Work out the finished part from the listing and answer in its coordinate system (mm). Face numbers are marked on the shaded views. Round coordinates to 2 decimals unless told otherwise and drop trailing zeros. Loops run counter-clockwise (first coordinate to the right, second up) from the corner with the lowest first, then second, coordinate; pieces in that order, holes last. Notation, with made-up numbers: (61, 53.5) -> (89, 53.5) arc R21 ccw to (89, 82.5) -> close; hole circle Ø1 at (-39, -37.5). An arc over 180 degrees is marked (long way). Write item = value, one per line. Start each with the question number.
```python
from build123d import *

# Parameters (mm, degrees)
F0_W     = 900
F0_H     = 2000
F1_DEPTH = 270
F2_R     = 20
F3_W     = 80
F3_H     = 80
F4_DEPTH = 100


with BuildPart() as f1:
    # F0 (on Top) → F1 (new body)
    with BuildSketch(Plane.XY):
        Rectangle(F0_W, F0_H)
    extrude(amount=F1_DEPTH)

    # F2
    f2_edges = [f1.edges().sort_by_distance(p)[0] for p in [
        (-450, 0, 270),
        (0, 1000, 270),
        (450, 0, 270),
        (0, -1000, 270),
        (450, -1000, 135),
        (450, 1000, 135),
        (-450, 1000, 135),
        (-450, -1000, 135),
    ]]
    fillet(f2_edges, radius=F2_R)

    # F3 (on face) → F4 (join)
    with BuildSketch(Plane(origin=(0, 0, 0), x_dir=(1, 0, 0), z_dir=(0, 0, -1))):
        with Locations((-400, 780)):
            Rectangle(F3_W, F3_H)
        with Locations((400, 780)):
            Rectangle(F3_W, F3_H)
        with Locations((400, -780)):
            Rectangle(F3_W, F3_H)
        with Locations((-400, -780)):
            Rectangle(F3_W, F3_H)
    extrude(amount=F4_DEPTH)


solid = f1.part
```
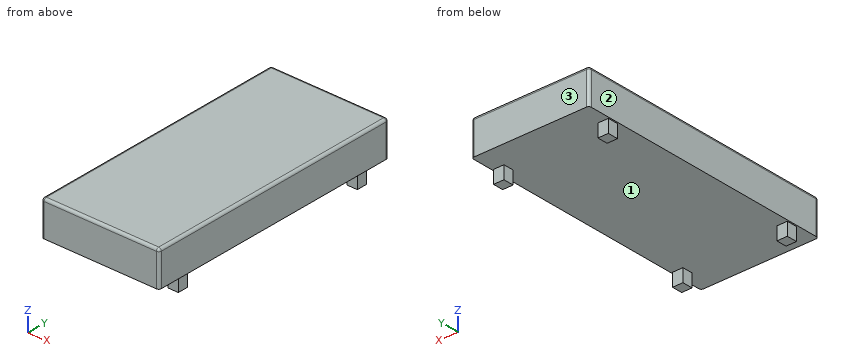
Item 1: Section B-B (y = -795) is taken. Determine the outline of the cut face in (x, z), then the cut area to 3 significant figures.
Item 2: Flat-ended cylindrical pins translate along their axes: pin 1 (1.5 mm diameter, centred on x = -15, y = -254.5, fed in from -Z); pin 2 (24 mm diameter, centred on y = 782.5, z = -72.5, fed in from +X); pin 3 (24 mm diameter, centred on y = 774.5, z = -49.5, fed in from -X). Find the tip coordinate at first contact, or state that the pin passes through.
Item 3: Find the intervals of material crossed by line 1 along Y through (x, z) = (409.5, -20); line 2 along Z through (x, y) = (341, -375), in increasing order. Write a range as [from, to].
Item 4: The mould has two halves that part along Y. Classify the marked faces 1, 2 and 3: pulls with the +Y half, pulls with the -Y half, needs draft (parallel to the pull), parting line crosses it, or undercut.
Item 5: Section C-C (x = 271) is taken. Determine the outline of the cut face in (y, z).
Item 6: Section A-A (z = -61) is taken. Determine the outline of the cut face in (x, y), then the cut area to 3 significant figures.
Item 7: Section D-D (y = 531) is taken. Determine the outline of the cut face in (x, z).
Worked answers:
q1.outline = (-450, 0) -> (-440, 0) -> (-440, -100) -> (-360, -100) -> (-360, 0) -> (360, 0) -> (360, -100) -> (440, -100) -> (440, 0) -> (450, 0) -> (450, 250) arc R20 ccw to (430, 270) -> (-430, 270) arc R20 ccw to (-450, 250) -> close
q1.area = 259,000 mm2
q2.pin_1 = 0
q2.pin_2 = 440
q2.pin_3 = -440
q3.line_1 = [-820, -740], [740, 820]
q3.line_2 = [0, 270]
q4.face_1 = undercut
q4.face_2 = needs draft
q4.face_3 = pulls with the +Y half
q5.outline = (-1000, 0) -> (1000, 0) -> (1000, 250) arc R20 ccw to (980, 270) -> (-980, 270) arc R20 ccw to (-1000, 250) -> close
q6.outline = (-440, -820) -> (-360, -820) -> (-360, -740) -> (-440, -740) -> close; (-440, 740) -> (-360, 740) -> (-360, 820) -> (-440, 820) -> close; (360, -820) -> (440, -820) -> (440, -740) -> (360, -740) -> close; (360, 740) -> (440, 740) -> (440, 820) -> (360, 820) -> close
q6.area = 25,600 mm2
q7.outline = (-450, 0) -> (450, 0) -> (450, 250) arc R20 ccw to (430, 270) -> (-430, 270) arc R20 ccw to (-450, 250) -> close
